Design review of the part built by this model. Coordinates are the model's own, in mm. Round coordinates to 2 decimals unless told otherwise and drop trailing zeros. Write each loop counter-clockwise with the first axis right and the second up, starting at its lowest first coordinate (ties: lowest second). Pieces come first, ordered by that corner, then holes. Notation, with made-up numbers: (2.25, 83.5) -> (50.25, 83.5) arc R22 ccw to (50.25, 103.5) -> close; hole circle Ø11 at (73, -19). An arc over 180 degrees is marked (long way). Write item = value, one per line. Start each with the question number.
Item 1: Add section B-B, the plane z = -6. State the section outline as (x, y) points, then the cut area to 3 significant figures.
Item 2: To check wall thickness, follow L1, parallel to Y at x = 20, z = 0; L2, parallel to X at y = 139, z = 0; L3, parallel to Z at x = -4.5, y = 106. State the ranges of each line that lie inside material, in increasing order.
Item 3: For pin 1 Ø4 at (y, z) = (22.225, 0) entering from +X; pin 2 Ø8 at (y, z) = (121.44, 0) entering from +X; pin 3 Ø1 at (x, y) = (7, 70) entering from -Z; pin 4 Ø1 at (y, z) = (34, 2.5) entering from -X, all flat-tipped, find the tip position at first contact; note any pin that passes through.
Item 4: Add section C-C, the plane y = 160. State the section outline as (x, z) points, then the cut area to 3 significant figures.
Item 5: Mouldability with a two-part tool opening along Y and no side actions: class faces 1 (the cylindrical face through (-19.191, 19.826, 0.533)), 2 (the flat face through (-16, 304.8, 8)), 3 (the flat face through (-16, 0, 8)), 4 (the cylindrical face through (10.66, 150.27, 13.91)) as released by +Y, released by -Y, zero draft, split by the parting line, or undercut.
Item 6: Add section A-A, the plane x = 0. State the section outline as (y, z) points, then the cut area to 3 significant figures.
from build123d import *

# Parameters (mm, degrees)
SKETCH1_R                    = 21.082
SKETCH1_R_2                  = 17.526
BOSS_EXTRUDE1_DEPTH          = 304.8
F_10_0_1935_DIAMETER_HOLE1_D = 4.9149
F_1_4_CLEARANCE_HOLE1_D      = 6.7564


with BuildPart() as part:
    # Sketch1 → Boss-Extrude1 (new body)
    with BuildSketch(Plane(origin=(0, 0, 0), x_dir=(1, 0, 0), z_dir=(0, 1, 0))):
        with Locations(Location((0, 0, 0), (0, 0, 90))):
            Circle(SKETCH1_R)
        with Locations(Location((0, 0, 0), (0, 0, 90))):
            Circle(SKETCH1_R_2, mode=Mode.SUBTRACT)
    extrude(amount=BOSS_EXTRUDE1_DEPTH)

    # #10 (0.1935) Diameter Hole1 (through all)
    with Locations(Plane.ZY.offset(21.082)):
        with Locations((0, 22.225), (0, 60.325)):
            Hole(F_10_0_1935_DIAMETER_HOLE1_D / 2)

    # 1/4 Clearance Hole1 (through all)
    with Locations(Plane(origin=(-21.082, 0, 0), x_dir=(0, 0, -1), z_dir=(-1, 0, 0))):
        with Locations((0, -121.44375)):
            Hole(F_1_4_CLEARANCE_HOLE1_D / 2)


solid = part.part
Result set:
q1.outline = (-20.21, 0) -> (-16.47, 0) -> (-16.47, 304.8) -> (-20.21, 304.8) -> close; (16.47, 0) -> (20.21, 0) -> (20.21, 304.8) -> (16.47, 304.8) -> close
q1.area = 2,280 mm²
q2.L1 = 0 to 19.77, 24.68 to 57.87, 62.78 to 118.07, 124.82 to 304.8
q2.L2 = -21.08 to -17.53, 17.53 to 21.08
q2.L3 = -20.6 to -16.94, 16.94 to 20.6
q3.pin_1 = through
q3.pin_2 = 21.08
q3.pin_3 = -20.05
q3.pin_4 = -20.99
q4.outline = circle Ø42.16 at (0, 0); hole circle Ø35.05 at (0, 0)
q4.area = 431 mm²
q5.face_1 = undercut
q5.face_2 = released by +Y
q5.face_3 = released by -Y
q5.face_4 = zero draft
q6.outline = (0, -21.08) -> (304.8, -21.08) -> (304.8, -17.53) -> (0, -17.53) -> close; (0, 17.53) -> (304.8, 17.53) -> (304.8, 21.08) -> (0, 21.08) -> close
q6.area = 2,170 mm²
